```python
from build123d import *

# Parameters (mm, degrees)
BOSS_EXTRUDE1_DEPTH = 10
SKETCH2_W           = 5.8
SKETCH2_H           = 3.8
BOSS_EXTRUDE2_DEPTH = 2
SKETCH3_R           = 2.15
CUT_EXTRUDE1_DEPTH  = 12
CUT_EXTRUDE2_DEPTH  = 6.5
SKETCH5_W           = 7.6
SKETCH5_H           = 3.5
CUT_EXTRUDE3_DEPTH  = 6.5
SKETCH6_R           = 2.15
CUT_EXTRUDE4_DEPTH  = 7.3
CUT_EXTRUDE5_START  = -10
CUT_EXTRUDE5_DEPTH  = 7.5
SKETCH8_W           = 7.6
SKETCH8_H           = 3.5
CUT_EXTRUDE6_DEPTH  = 8.75


with BuildPart() as part:
    # Sketch1 → Boss-Extrude1 (new body)
    with BuildSketch(Plane.XY):
        Polygon((0, 70.768728377), (0, 0), (33, 0), align=None)
    extrude(amount=BOSS_EXTRUDE1_DEPTH)

    # Sketch2 → Boss-Extrude2 (add)
    with BuildSketch(Plane(origin=(0, 0, 0), x_dir=(-1, 0, 0), z_dir=(0, -1, 0))):
        with Locations((-16.5, -5)):
            Rectangle(SKETCH2_W, SKETCH2_H)
    extrude(amount=BOSS_EXTRUDE2_DEPTH)

    # Sketch3 → Cut-Extrude1 (cut)
    with BuildSketch(Plane(origin=(0, 0, 0), x_dir=(-1, 0, 0), z_dir=(0, -1, 0))):
        with Locations(Location((-23.331538291, -4, 0), (0, 0, 180))):
            Circle(SKETCH3_R)
        with Locations(Location((-8.551538291, -4, 0), (0, 0, 180))):
            Circle(SKETCH3_R)
    extrude(amount=-CUT_EXTRUDE1_DEPTH, mode=Mode.SUBTRACT)

    # Sketch4 → Cut-Extrude2 (cut)
    with BuildSketch(Plane(origin=(0, 0, 0), x_dir=(-1, 0, 0), z_dir=(0, 0, -1))):
        Polygon((-19.531538291, 3.25), (-19.531538291, 5), (-19.531538291, 6.75), (-27.131538291, 6.75), (-27.131538291, 5), (-27.131538291, 3.25), align=None)
    extrude(amount=-CUT_EXTRUDE2_DEPTH, mode=Mode.SUBTRACT)

    # Sketch5 → Cut-Extrude3 (cut)
    with BuildSketch(Plane(origin=(0, 0, 0), x_dir=(-1, 0, 0), z_dir=(0, 0, -1))):
        with Locations((-23.331538291, 5)):
            Rectangle(SKETCH5_W, SKETCH5_H)
        with Locations((-8.551538291, 5)):
            Rectangle(SKETCH5_W, SKETCH5_H)
    extrude(amount=-CUT_EXTRUDE3_DEPTH, mode=Mode.SUBTRACT)

    # Sketch6 → Cut-Extrude4 (cut)
    with BuildSketch(Plane(origin=(27.10599556, 12.639733311, 0), x_dir=(0, 0, -1), z_dir=(0.9063077870366479, 0.422618261740704, 0))):
        with Locations(Location((-5, 9.053597363, 0), (0, 0, 90))):
            Circle(SKETCH6_R)
        with Locations(Location((-5, 39.053597363, 0), (0, 0, 90))):
            Circle(SKETCH6_R)
    extrude(amount=-CUT_EXTRUDE4_DEPTH, mode=Mode.SUBTRACT)

    # Sketch7 → Cut-Extrude5 (cut)
    with BuildSketch(Plane.XY.offset(10).offset(CUT_EXTRUDE5_START)):
        Polygon((6.247556837, 50.199361906), (3.358673988, 48.823005888), (6.627519532, 41.961909123), (9.51640238, 43.338265141), align=None)
        Polygon((18.982454602, 23.03825064), (22.13718624, 16.123941687), (19.225898259, 14.795633629), (16.071166622, 21.709942582), align=None)
    extrude(amount=CUT_EXTRUDE5_DEPTH, mode=Mode.SUBTRACT)

    # Sketch8 → Cut-Extrude6 (cut)
    with BuildSketch(Plane(origin=(0, 0, 0), x_dir=(-1, 0, 0), z_dir=(0, 0, -1))):
        with Locations((-23.331538291, 5)):
            Rectangle(SKETCH8_W, SKETCH8_H)
        with Locations((-8.551538291, 5)):
            Rectangle(SKETCH8_W, SKETCH8_H)
        Polygon((-22.13718624, 16.123941687), (-19.225898259, 14.795633629), (-16.071166622, 21.709942582), (-18.982454602, 23.03825064), align=None)
        Polygon((-9.51640238, 43.338265141), (-6.627519532, 41.961909123), (-3.358673988, 48.823005888), (-6.247556837, 50.199361906), align=None)
    extrude(amount=-CUT_EXTRUDE6_DEPTH, mode=Mode.SUBTRACT)


solid = part.part
```
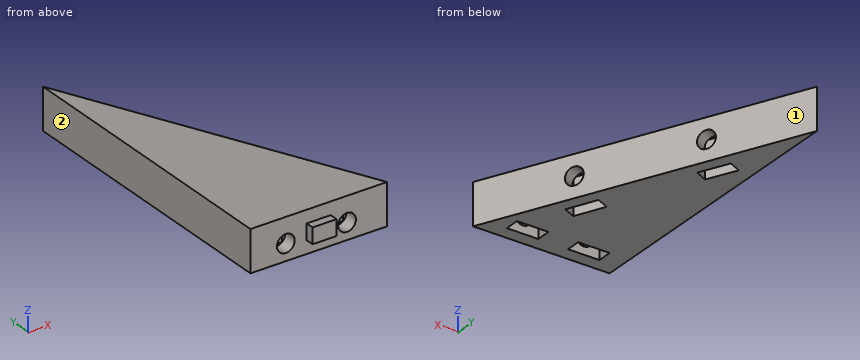
Geometry: final body of the model. Coordinates: model frame, mm. Face numbers are marked on the shaded views. Round coordinates to 2 decimals unless told otherwise and drop trailing zeros. Order: outer loops, then holes, each group sorted by start corner. A loop starts at its lowest first (then second) coordinate and runs counter-clockwise, first axis right, second up. Notation, with made-up numbers: M 75,8.5 L 134,8.5 A31 ccw 134,45.5 Z; hole C -21,-36.5 d9. An arc over 180 degrees is marked long. Use one line per item in the form item = value. Start each with the question number.
Q1. Cut plane C-C (y = 54). Return loops of the section in (x, z).
Q2. Mould query, pull axis Y, two halves, no side actions, for the marked faces 1 and 2. Classes: +Y half, -Y half, draft (parallel to the pull), parting line (faces both ways), or undercut.
Q3. Pin query (flat end, axial travel): pin 1 Ø4 at (x, z) = (23.5, 6) entering from +Y; pin 2 Ø6 at (x, z) = (9, 3) entering from +Y; pin 3 Ø3 at (y, z) = (18, 6.5) entering from +X. Return the tip coordinate at first contact, or that it passes through.
Q4. Material intervals for line 1 (X direction, y = 4, z = 6.5); line 2 (Y direction, x = 21, z = 2.5); line 3 (Z direction, x = 10, y = 6), sorted ascending. Write a range as [from, to].
Q5. Cut plane A-A (z = 8). Return loops of the section in (x, y), and give its area (3 significant figures).
Q6. Cut plane B-B (x = 31). Return loops of the section in (y, z), and give its area (3 significant figures).
Geometry results:
q1.outline = M 0,0 L 7.82,0 L 7.82,10 L 0,10 Z
q2.face_1 = +Y half
q2.face_2 = draft
q3.pin_1 = 24.66
q3.pin_2 = 57.9
q3.pin_3 = 25.31
q4.line_1 = [0, 4.75], [12.35, 19.53], [27.13, 31.13]
q4.line_2 = [0, 3.25], [6.75, 15.61], [18.62, 25.73]
q4.line_3 = [8.75, 10]
q5.outline = M 0,0 L 33,0 L 0,70.77 Z; hole M 3.36,48.82 L 6.63,41.96 L 9.52,43.34 L 6.25,50.2 Z; hole M 4.75,3.25 L 12.35,3.25 L 12.35,6.75 L 4.75,6.75 Z; hole M 16.07,21.71 L 19.23,14.8 L 22.14,16.12 L 18.98,23.04 Z; hole M 19.53,3.25 L 27.13,3.25 L 27.13,6.75 L 19.53,6.75 Z
q5.area = 1,070 mm^2
q6.outline = M 0,0 L 4.29,0 L 4.29,10 L 0,10 Z
q6.area = 42.9 mm^2
